```python
from build123d import *

# Parameters (mm, degrees)
SKETCH1_W           = 28
SKETCH1_H           = 56.5
BOSS_EXTRUDE1_DEPTH = 30
CUT_EXTRUDE2_DEPTH  = 56.5
SHELL1_T            = -1
BOSS_EXTRUDE3_DEPTH = 2.5
SKETCH4_R           = 0.35
CUT_EXTRUDE1_DEPTH  = 5
BOSS_EXTRUDE4_DEPTH = 56.5
BOSS_EXTRUDE5_START = -11.087816
SKETCH7_R           = 8.5
BOSS_EXTRUDE5_DEPTH = 11.087816
SKETCH8_R           = 7
CUT_EXTRUDE3_DEPTH  = 2
LPATTERN1_COUNT     = 2
LPATTERN1_PITCH     = 20


with BuildPart() as part:
    # Sketch1 → Boss-Extrude1 (new body)
    with BuildSketch(Plane(origin=(0, 0, 0), x_dir=(1, 0, 0), z_dir=(0, 1, 0))):
        Rectangle(SKETCH1_W, SKETCH1_H)
    extrude(amount=-BOSS_EXTRUDE1_DEPTH)

    # Sketch5 → Cut-Extrude2 (cut)
    with BuildSketch(Plane(origin=(0, 0, -28.25), x_dir=(-1, 0, 0), z_dir=(0, 0, -1))):
        with BuildLine():
            Line((-1, -30), (-1, -26))
            ThreePointArc((-1, -26), (3.188611699, -13.752551286), (14, -6.635083269))
            Line((14, -6.635083269), (14, -30))
            Line((14, -30), (-1, -30))
        make_face()
    extrude(amount=-CUT_EXTRUDE2_DEPTH, mode=Mode.SUBTRACT)

    # Shell1
    shell1_openings = [part.faces().sort_by_distance(p)[0] for p in [
        (7.5, -30, 0),
        (0.885231383, -15.011682153, -28.25),
        (-4.84430585, -15.03504646, 0),
        (1, -28, 0),
    ]]
    offset(amount=SHELL1_T, openings=shell1_openings, kind=Kind.INTERSECTION)

    # Sketch3 → Boss-Extrude3 (add, symmetric)
    with BuildSketch(Plane.XY.offset(-20)):
        with BuildLine():
            Line((-14, -1), (-15, -1))
            ThreePointArc((-15, -1), (-15.5, -1.5), (-15, -2))
            Line((-15, -2), (-14, -2))
            Line((-14, -2), (-12.5, -1))
            Line((-12.5, -1), (-14, -1))
        make_face()
    boss_extrude3 = extrude(amount=BOSS_EXTRUDE3_DEPTH, both=True)

    # Sketch4 → Cut-Extrude1 (cut)
    with BuildSketch(Plane(origin=(0, 0, -22.5), x_dir=(-1, 0, 0), z_dir=(0, 0, -1))):
        with Locations((15, -1.5)):
            Circle(SKETCH4_R)
    cut_extrude1 = extrude(amount=-CUT_EXTRUDE1_DEPTH, mode=Mode.SUBTRACT)

    # Mirror1: Boss-Extrude3, Cut-Extrude1 across plane
    add(boss_extrude3.mirror(Plane.XY))
    add(cut_extrude1.mirror(Plane.XY), mode=Mode.SUBTRACT)

    # Sketch6 → Boss-Extrude4 (add)
    with BuildSketch(Plane(origin=(0, 0, -28.25), x_dir=(-1, 0, 0), z_dir=(0, 0, -1))):
        Polygon((-30, -3.677832944), (-21, -25), (-14, -30), (-14, 0), align=None)
        with BuildLine():
            Line((14, 0), (14, 2.5))
            ThreePointArc((14, 2.5), (-0.085690207, 2.209730318), (-14, 0))
            Line((-14, 0), (14, 0))
        make_face()
    extrude(amount=-BOSS_EXTRUDE4_DEPTH)

    # Sketch7 → Boss-Extrude5 (add)
    with BuildSketch(Plane(origin=(33, 0, 0), x_dir=(0, 0, -1), z_dir=(1, 0, 0)).offset(BOSS_EXTRUDE5_START)):
        with Locations((10.25, -14.338916472)):
            Circle(SKETCH7_R)
    boss_extrude5 = extrude(amount=BOSS_EXTRUDE5_DEPTH)

    # Sketch8 → Cut-Extrude3 (cut)
    with BuildSketch(Plane(origin=(33, 0, 0), x_dir=(0, 0, -1), z_dir=(1, 0, 0))):
        with Locations((10.25, -14.338916472)):
            Circle(SKETCH8_R)
    cut_extrude3 = extrude(amount=-CUT_EXTRUDE3_DEPTH, mode=Mode.SUBTRACT)

    # LPattern1: Boss-Extrude5, Cut-Extrude3 ×2
    with Locations(*[(0, 0, i * LPATTERN1_PITCH) for i in range(1, LPATTERN1_COUNT)]):
        add(boss_extrude5)
        add(cut_extrude3, mode=Mode.SUBTRACT)


solid = part.part
```
Part model, mm, in its own coordinate system. A direction names the side the tool comes from. Give positions to 0.01 mm unless a question says otherwise; leave off trailing zeros. Loops run counter-clockwise (first coordinate to the right, second up) from the corner with the lowest first, then second, coordinate; pieces in that order, holes last. Notation, with made-up numbers: M -39,-15.75 L -11,-15.75 A24 cw -11,-0.75 Z; hole C -36,-23 d9. An arc over 180 degrees is marked long. Return JSON: item names as keys, results as strings.
1) Saw through at D-D, the plane y = -27.5. List the corners of the cut face in (x, z), then the cut area to 3 significant figures.
Calculated:
{"outline": "M 1,27.25 L 13,27.25 L 13,-28.25 L 17.5,-28.25 L 17.5,28.25 L 1,28.25 Z", "area": "266 mm2"}
2) Pull direction Y, two halves, no side cores. Call faces 1 (the face through (31, -14, -10)), 2 (the face through (32.01, -12.24, -16.93)), 3 (the face through (33, -7, 9)), 4 (the face through (21.888, -1.813, -0.396)): released by +Y, released by -Y, zero draft, split by the parting line, or undercut.
Calculated:
{"face 1": "undercut", "face 2": "undercut", "face 3": "zero draft", "face 4": "released by +Y"}
3) Saw through at C-C, the plane x = 24.5. List the corners of the cut face in (y, z), then the cut area to 3 significant figures.
Calculated:
{"outline": "M -16.71,-28.25 L -2.41,-28.25 L -2.41,28.25 L -16.71,28.25 L -16.71,17.91 A8.5 ccw -16.71,1.59 L -16.71,-2.09 A8.5 ccw -16.71,-18.41 Z", "area": "955 mm2"}
4) Saw through at B-B, the plane y = -19. List the corners of the cut face in (x, z) (3 decimals), then the cut area to 3 significant figures.
Calculated:
{"outline": "M -0.265,27.25 L 13,27.25 L 13,-28.25 L 23.533,-28.25 L 23.533,-17.358 L 33,-17.358 L 33,-15.472 L 31,-15.472 L 31,-5.028 L 33,-5.028 L 33,-3.142 L 23.533,-3.142 L 23.533,2.642 L 33,2.642 L 33,4.528 L 31,4.528 L 31,14.972 L 33,14.972 L 33,16.858 L 23.533,16.858 L 23.533,28.25 L -0.265,28.25 Z", "area": "836 mm2"}
5) Saw through at A-A, the plane z = -10.25. List the corners of the cut face in (x, y).
Calculated:
{"outline": "M -14,-6.64 A20 cw -13,-6.92 L -13,-1 L 13,-1 L 13,-30 L 14,-30 L 21,-25 L 21.91,-22.84 L 33,-22.84 L 33,-21.34 L 31,-21.34 L 31,-7.34 L 33,-7.34 L 33,-5.84 L 29.09,-5.84 L 30,-3.68 L 14,0 A103 ccw -14,2.5 Z"}
6) 3-axis set-ups, long thin cutter, end or side, ignore diameter. For faces 5 (the face through (31, -14, 10)), 6 (the face through (-0.111, 2.227, -0.396)): which of +Z, -Z, +X, -X, +Y, -Y reach the whole face in a straight line?
Calculated:
{"face 5": "+X", "face 6": "+Z, -Z, +Y"}
7) Drill centre lines: line 1 (Y direction, x = -15, z = -18.8); line 2 (X direction, y = -14.5, z = -2.5); line 3 (Z direction, x = 11, y = -18). Where is each one in solid material? Low to high.
Calculated:
{"line 1": "y = -2 to -1.85, -1.15 to -1", "line 2": "x = 13 to 33", "line 3": "z = 27.25 to 28.25"}
8) Flat gauge pins, fed straight in: pin 1 Ø1.1 at (x, y) = (-15, -1.5) entering from -Z; pin 2 Ø5 at (x, z) = (26.5, -17.5) entering from -Y; pin 3 Ø1 at (y, z) = (-11.5, -2) entering from -X. Where does each tip first touch, or does it go through?
Calculated:
{"pin 1": "stops at z = -22.5", "pin 2": "stops at y = -21.39", "pin 3": "stops at x = 13"}
